```python
from build123d import *

# Parameters (mm, degrees)
F0_R        = 8.925
F1_DEPTH    = 45
F2_R        = 6
F3_DEPTH    = 40
F4_R        = 10.25
F4_R_2      = 8.925
F5_DEPTH    = 1.5
F6_S5_R     = 8.925
F6_T6_DEPTH = 16


# Not quite as in the source:
# - a fillet or chamfer that OpenCascade refuses, or shapes differently, is made with other operations: its cross-section is extruded or revolved along the edge and cut away or added


with BuildPart() as f1:
    # F0 (on Top) → F1 (new body)
    with BuildSketch(Plane.XY):
        Circle(F0_R)
    extrude(amount=F1_DEPTH)

    # F2 (on face) → F3 (cut)
    with BuildSketch(Plane.XY.offset(45)):
        Circle(F2_R)
    extrude(amount=-F3_DEPTH, mode=Mode.SUBTRACT)

    # F4 (on face) → F5 (join)
    with BuildSketch(Plane.XY.offset(45)):
        Circle(F4_R)
        Circle(F4_R_2, mode=Mode.SUBTRACT)
    extrude(amount=-F5_DEPTH)

    # F6: chamfer of 1.5 on 1 edges, made by hand


with BuildPart() as f6_tool2:
    # F6_s3 → F6_t4 (revolve)
    with BuildSketch(Plane.XZ):
        Polygon((8.75, 43.5), (10.25, 45), (10.25, 43.5), align=None)
    revolve(axis=Axis((0, 0, 43.5), (0, 0, 1)))

    # F6_s5 → F6_t6 (cut, symmetric)
    with BuildSketch(Plane.XY.offset(44.2)):
        Circle(F6_S5_R)
    extrude(amount=F6_T6_DEPTH, both=True, mode=Mode.SUBTRACT)


with BuildPart() as f1_1:
    add(f1.part)

    # F6_t1: cut F6_tool2
    add(f6_tool2.part, mode=Mode.SUBTRACT)


solid = f1_1.part
```
Build history of the part. All positions in model axes, mm. A direction names the side the tool comes from. Round coordinates to 2 decimals unless told otherwise and drop trailing zeros. Write each loop counter-clockwise with the first axis right and the second up, starting at its lowest first coordinate (ties: lowest second). Pieces come first, ordered by that corner, then holes. Notation, with made-up numbers: (9.5, 71.25) -> (49.5, 71.25) arc R18 cw to (49.5, 81.25) -> close; hole circle Ø2 at (11.25, 88.25). An arc over 180 degrees is marked (long way). Put each result on its own line as item: value.
Item 1: Two-plate mould, pull along Y, no slides. Class faces 1 (the face through (-6, 0, 25)), 2 (the face through (-1.935, -8.713, 22.143)), 3 (the face through (4.4, -4.4, 45)): pulls with the +Y half, pulls with the -Y half, needs draft (parallel to the pull), parting line crosses it, or undercut.
Here are the results:
face 1: undercut
face 2: parting line crosses it
face 3: needs draft
Item 2: Wall check: probe 1 along Y at (x, z) = (0, 21.5) (3 decimals); probe 2 along Z at (x, y) = (-3.25, -4.25); probe 3 along Y at (x, z) = (1, 14.5). Give the ranges that are in metal, low to high. Write a range as from..to.
Here are the results:
probe 1: y = -8.925..-6, 6..8.925
probe 2: z = 0..5
probe 3: y = -8.87..-5.92, 5.92..8.87
Item 3: Flat gauge pins, fed straight in: P1, Ø1, axis at y = -3.5, z = 20.5, coming from the +X side; P2, Ø12, axis at x = -5.5, z = 13, coming from the -Y side (3 decimals); P3, Ø10, axis at y = -3.5, z = 21, coming from the +X side (3 decimals). Where does each tip first touch, or does it go through?
Here are the results:
P1: stops at x = 8.41
P2: stops at y = -8.925
P3: stops at x = 8.925
Item 4: Slice it at C-C, the plane z = 21.5. Give the cut face in (x, y) (3 decimals), plus the area to 3 significant figures.
Here are the results:
outline: circle Ø17.85 at (0, 0); hole circle Ø12 at (0, 0)
area: 137 mm^2
Item 5: Tool access for faces 4 (the face through (0, 0, 5)), 5 (the face through (0, 0, 0)): list every direction of +Z, -Z, +X, -X, +Y, -Y with a clear straight run to the whole face (end or side of a thin tool).
Here are the results:
face 4: +Z
face 5: -Z, +X, -X, +Y, -Y
Item 6: Slice it at A-A, the plane x = 0. Give the cut face in (y, z) (3 decimals).
Here are the results:
outline: (-10.25, 45) -> (-8.925, 43.675) -> (-8.925, 0) -> (8.925, 0) -> (8.925, 43.675) -> (10.25, 45) -> (6, 45) -> (6, 5) -> (-6, 5) -> (-6, 45) -> close
